Design review of the part built by this model. Coordinates are the model's own, in mm. A direction names the side the tool comes from. Coordinates: 2 decimals unless noted, no trailing zeros. Loops run counter-clockwise (first coordinate to the right, second up) from the corner with the lowest first, then second, coordinate; pieces in that order, holes last. Notation, with made-up numbers: M 23.5,-37 L 67.5,-37 A19 ccw 67.5,-23 Z; hole C 76,81.25 d3. An arc over 180 degrees is marked long. One line per item, written item: value.
```python
from build123d import *

# Parameters (mm, degrees)
SKETCH1_R                 = 10
SKETCH1_R_2               = 6.25
COLLAR_RING_DEPTH         = 9
SKETCH2_W                 = 7
SKETCH2_H                 = 9
SCREW_BOSS_DEPTH          = 9
SKETCH3_R                 = 1.3
M3_THUMB_SCREW_HOLE_DEPTH = 5.5


with BuildPart() as part:
    # Sketch1 → Collar_ring (new body)
    with BuildSketch(Plane.XY):
        Circle(SKETCH1_R)
        Circle(SKETCH1_R_2, mode=Mode.SUBTRACT)
    extrude(amount=COLLAR_RING_DEPTH)

    # Sketch2 → Screw_boss (add)
    with BuildSketch(Plane.XY):
        with Locations((11.5, 0)):
            Rectangle(SKETCH2_W, SKETCH2_H)
    extrude(amount=SCREW_BOSS_DEPTH)

    # Sketch3 → M3_thumb_screw_hole (cut, symmetric)
    with BuildSketch(Plane(origin=(10.5, 0, 0), x_dir=(0, 0, -1), z_dir=(1, 0, 0))):
        with Locations(Location((-4.5, 0, 0), (0, 0, 180))):
            Circle(SKETCH3_R)
    extrude(amount=M3_THUMB_SCREW_HOLE_DEPTH, both=True, mode=Mode.SUBTRACT)


solid = part.part
```
(1) Mouldability with a two-part tool opening along Z and no side actions: class faces 1 (the cylindrical face through (10.62, -0.39, 5.74)), 2 (the flat face through (5, -4, 9)), 3 (the cylindrical face through (-10, 0, 4)) as released by +Z, released by -Z, zero draft, split by the parting line, or undercut.
Reply:
face 1: undercut
face 2: released by +Z
face 3: zero draft
(2) We need section C-C on z = 4.5. State the section outline as (x, y) points, then the cut area to 3 significant figures.
Reply:
outline: M 6.11,-1.3 A6.25 cw long 6.11,1.3 L 15,1.3 L 15,4.5 L 8.93,4.5 A10 ccw long 8.93,-4.5 L 15,-4.5 L 15,-1.3 Z
area: 217 mm2
(3) We need section D-D on x = 12.5. State the section outline as (y, z) points, then the cut area to 3 significant figures.
Reply:
outline: M -4.5,0 L 4.5,0 L 4.5,9 L -4.5,9 Z; hole C 0,4.5 d2.6
area: 75.7 mm2
(4) We need section A-A on x = 0. State the section outline as (y, z) points, then the cut area to 3 significant figures.
Reply:
outline: M -10,0 L -6.25,0 L -6.25,9 L -10,9 Z; M 6.25,0 L 10,0 L 10,9 L 6.25,9 Z
area: 67.5 mm2
(5) We need section B-B on y = 0. State the section outline as (x, z) points, then the cut area to 4 significant figures.
Reply:
outline: M -10,0 L -6.25,0 L -6.25,9 L -10,9 Z; M 6.25,0 L 15,0 L 15,3.2 L 6.25,3.2 Z; M 6.25,5.8 L 15,5.8 L 15,9 L 6.25,9 Z
area: 89.75 mm2
(6) To check wall thickness, follow line 1 along Y through (x, z) = (0, 5.5); line 2 along Y through (x, z) = (11.5, 4.5); line 3 along Y through (x, z) = (12.5, 1). State the ranges of each line that lie inside material, in increasing order. Write a range as [from, to].
Reply:
line 1: y = [-10, -6.25], [6.25, 10]
line 2: y = [-4.5, -1.3], [1.3, 4.5]
line 3: y = [-4.5, 4.5]
(7) Insertion check: pin 1 (1 mm diameter, centred on x = 9, y = -1, fed in from -Z); pin 2 (5 mm diameter, centred on y = 7.5, z = 7, fed in from +X); pin 3 (3 mm diameter, centred on x = 11.5, z = 5.5, fed in from -Y); pin 4 (1.8 mm diameter, centred on x = 12, z = 6, fed in from +Y). Each pin has a flat end and moves straight along its axis. Give the tip position at first contact, or say it passes through.
Reply:
pin 1: stops at z = 0
pin 2: stops at x = 8.66
pin 3: stops at y = -4.5
pin 4: stops at y = 4.5
(8) Tool access review of faces 4 (the flat face through (12, -4.5, 4)), 5 (the flat face through (12, 4.5, 4)), 6 (the flat face through (5, -4, 0)): name each direction out of +Z, -Z, +X, -X, +Y, -Y from which nothing blocks a thin tool from reaching the whole face with its end or side.
Reply:
face 4: +Z, -Z, +X, -Y
face 5: +Z, -Z, +X, +Y
face 6: -Z, +X, -X, +Y, -Y
